Design review of the part built by this model. Coordinates are the model's own, in mm. A direction names the side the tool comes from. Give positions to 0.01 mm unless a question says otherwise; leave off trailing zeros. Write each loop counter-clockwise with the first axis right and the second up, starting at its lowest first coordinate (ties: lowest second). Pieces come first, ordered by that corner, then holes. Notation, with made-up numbers: M 14,86.25 L 72,86.25 A29 cw 72,107.25 Z; hole C 46,83.5 d4. An arc over 180 degrees is marked long. Write each question's results on one line, items separated by ' | '. Start each with the question number.
from build123d import *

# Parameters (mm, degrees)
F1_DEPTH = 5.603792


with BuildPart() as f1:
    # F0 (on Front) → F1 (new body)
    with BuildSketch(Plane.XZ):
        Polygon((0, -7.449928), (0, 0), (-68.460882, -68.272778), (-75.931335, -75.722706), (-68.460882, -75.722706), align=None)
        Polygon((75.306922, 0), (67.83846, 0), (67.83846, -68.025367), (75.306922, -75.514406), align=None)
        Polygon((-75.931335, -75.722706), (-68.460882, -68.272778), (-68.460882, 0), (-75.931335, 0), align=None)
        Polygon((67.83846, -68.025367), (0, 0), (0, -7.449928), (68.484643, -76.123258), (75.306922, -75.514406), align=None)
    extrude(amount=F1_DEPTH)


solid = f1.part
Q1. Wall thickness on line 1 along X through (y, z) = (-1.5, -14); line 2 along X through (y, z) = (-1.6, -8.5); line 3 along X through (y, z) = (-1.95, -72): over which ranges is each line inside the solid? List them lowest first. Write a range as from..to.
Q2. For pin 1 Ø1 at (x, y) = (51.5, -4.5) entering from -Z; pin 2 Ø3 at (x, y) = (-72, -4) entering from -Z, all flat-tipped, find the tip position at first contact; note any pin that passes through.
Q3. We need section C-C on x = 44. Write out the cut boundary in (y, z), and give its area (3 significant figures).
Q4. We need section B-B on z = -30.5. Write out the cut boundary in (x, y), and give its area (3 significant figures).
Q5. For faces 1 (the flat face through (-34.71, -2.763, -42.064)), 2 (the flat face through (-68.461, -3, -35)), 3 (the flat face through (-17, 0, -24)), list the 3-axis set-ups (+Z, -Z, +X, -X, +Y, -Y) from which the entire face can be reached by the end or side of a thin tool; tool diameter is ignored.
Q6. We need section A-A on y = -1.15. Write out the cut boundary in (x, z).
Q7. The part is to be moulded in two halves that separate along X. For faces 4 (the flat face through (-72, -3, -75.723)), 5 (the flat face through (67.838, -3, -34)), 6 (the flat face through (75.307, -3, -38)), 7 (the flat face through (34.394, -2.763, -34.489)), say which applies: pulls with the +X half, pulls with the -X half, needs draft (parallel to the pull), parting line crosses it, or undercut.
Answer sheet:
1) line 1: -75.93..-68.46, -14.04..-6.57, 6.53..13.96, 67.84..75.31 | line 2: -75.93..-68.46, -8.52..-1.05, 1.05..8.48, 67.84..75.31 | line 3: -75.93..-64.73, 64.37..75.31
2) pin 1: z = -59.59 | pin 2: z = -75.72
3) outline: M -5.6,-51.57 L 0,-51.57 L 0,-44.12 L -5.6,-44.12 Z | area: 41.7 mm^2
4) outline: M -75.93,-5.6 L -68.46,-5.6 L -68.46,0 L -75.93,0 Z; M -30.58,-5.6 L -23.11,-5.6 L -23.11,0 L -30.58,0 Z; M 22.99,-5.6 L 30.42,-5.6 L 30.42,0 L 22.99,0 Z; M 67.84,-5.6 L 75.31,-5.6 L 75.31,0 L 67.84,0 Z | area: 167 mm^2
5) face 1: -Z, +Y, -Y | face 2: +Z, +Y, -Y | face 3: +Z, -Z, +X, -X, +Y
6) outline: M -75.93,-75.72 L -68.46,-75.72 L 0,-7.45 L 68.48,-76.12 L 75.31,-75.51 L 75.31,0 L 67.84,0 L 67.84,-68.03 L 0,0 L -68.46,-68.27 L -68.46,0 L -75.93,0 Z
7) face 4: needs draft | face 5: undercut | face 6: pulls with the +X half | face 7: undercut
